```python
from build123d import *

# Parameters (mm, degrees)
SKETCH55_R               = 37
BOSS_EXTRUDE17_DEPTH     = 8
SKETCH56_R               = 37
SKETCH56_R_2             = 30
SKETCH56_R_3             = 28.8
CUT_EXTRUDE20_DEPTH      = 6
CUT_EXTRUDE21_DEPTH      = 5.5
FILLET1_R                = 0.5
FILLET2_R                = 2
BOSS_EXTRUDE18_START     = 6
BOSS_EXTRUDE18_DEPTH     = 6
CIRPATTERN1_COUNT        = 3
FILLET1_OF_CIRPATTERN1_R = 0.5
FILLET2_OF_CIRPATTERN1_R = 2


with BuildPart() as part:
    # Sketch55 → Boss-Extrude17 (new body)
    with BuildSketch(Plane.XY):
        Circle(SKETCH55_R)
        Polygon((-15.131119551888249, 22.33533974306702), (-25.90504070234881, -7.604599443277265), (-0.7697350404796751, -26.883764916532357), (25.354620105449243, -9.123888866834614), (16.52740298769779, 21.24243055544057), align=None, mode=Mode.SUBTRACT)
    extrude(amount=-BOSS_EXTRUDE17_DEPTH)

    # Sketch56 → Cut-Extrude20 (cut)
    # profile 1 of 2: a face of its own
    with BuildSketch(Plane.XY):
        Circle(SKETCH56_R)
        Circle(SKETCH56_R_2, mode=Mode.SUBTRACT)
    # profile 2 of 2: a face of its own
    with BuildSketch(Plane.XY):
        Circle(SKETCH56_R_3)
    extrude(amount=-CUT_EXTRUDE20_DEPTH, mode=Mode.SUBTRACT)

    # Sweep1: sweep along a path in Sketch58
    with BuildLine(Plane.XY.offset(-1)) as sweep1_path:
        ThreePointArc((32.05951496825865, -3.5), (32.25, 0), (32.05951496825865, 3.5))
    # Sketch59 → Sweep1 (sweep)
    with BuildSketch(Plane(origin=(0, 0, 0), x_dir=(1, 0, 0), z_dir=(0, 1, 0))):
        Polygon((32, 1.0000000000000009), (32, 4.6), (30, 5.25), (30, 1.0000000000000009), align=None)
    sweep1 = sweep(path=sweep1_path.line)

    # Sketch60 → Cut-Extrude21 (cut)
    with BuildSketch(Plane.XY):
        with BuildLine():
            Line((29.691011106511933, 4.294631471149185), (28.503370662251456, 4.122846212303217))
            ThreePointArc((28.503370662251456, 4.122846212303217), (28.570983048615947, 3.624765873225473), (28.629892436770504, 3.125581395348848))
            Line((28.629892436770504, 3.125581395348848), (29.822804621635946, 3.255813953488383))
            ThreePointArc((29.822804621635946, 3.255813953488383), (29.761440675641612, 3.7757977846098676), (29.691011106511933, 4.294631471149185))
        make_face()
        with BuildLine():
            Line((29.822804621635946, -3.255813953488384), (28.629892436770504, -3.1255813953488487))
            ThreePointArc((28.629892436770504, -3.1255813953488487), (28.57098304861595, -3.6247658732254733), (28.503370662251456, -4.122846212303217))
            Line((28.503370662251456, -4.122846212303217), (29.691011106511933, -4.294631471149185))
            ThreePointArc((29.691011106511933, -4.294631471149185), (29.761440675641612, -3.7757977846098676), (29.822804621635946, -3.255813953488384))
        make_face()
    cut_extrude21 = extrude(amount=-CUT_EXTRUDE21_DEPTH, mode=Mode.SUBTRACT)

    # Fillet1
    fillet1_edges = [part.edges().sort_by_distance(p)[0] for p in [
        (31.810991596411686, 3.472868217054266, -2.8000000000000003),
    ]]
    fillet(fillet1_edges, radius=FILLET1_R)

    # Fillet2
    fillet2_edges = [part.edges().sort_by_distance(p)[0] for p in [
        (31.810991596411686, -3.4728682170542657, -2.8000000000000003),
    ]]
    fillet(fillet2_edges, radius=FILLET2_R)

    # Sketch62 → Boss-Extrude18 (add)
    with BuildSketch(Plane.XY.offset(-6).offset(BOSS_EXTRUDE18_START)):
        with BuildLine():
            Line((35.035393105684086, 5.067665135956038), (28.225251300389694, 5.724961923877751))
            ThreePointArc((28.225251300389694, 5.724961923877751), (28.092883468127496, 6.342704348005581), (27.946997326196957, 6.957394659607891))
            Line((27.946997326196957, 6.957394659607891), (34.836258824834346, 6.29246144915893))
            ThreePointArc((34.836258824834346, 6.29246144915893), (34.94119298731927, 5.680935893223171), (35.035393105684086, 5.067665135956038))
        make_face()
    boss_extrude18 = extrude(amount=-BOSS_EXTRUDE18_DEPTH)

    # CirPattern1: Sweep1, Cut-Extrude21, Boss-Extrude18 ×3 about axis
    cirpattern1_axis = Axis((-3.9e-16, -9.2e-16, 0), (0, 0, 1))
    add([sweep1.rotate(cirpattern1_axis, i * 360 / CIRPATTERN1_COUNT) for i in range(1, CIRPATTERN1_COUNT)])
    add([cut_extrude21.rotate(cirpattern1_axis, i * 360 / CIRPATTERN1_COUNT) for i in range(1, CIRPATTERN1_COUNT)], mode=Mode.SUBTRACT)
    add([boss_extrude18.rotate(cirpattern1_axis, i * 360 / CIRPATTERN1_COUNT) for i in range(1, CIRPATTERN1_COUNT)])

    # Fillet1 of CirPattern1
    fillet1_of_cirpattern1_edges = [part.edges().sort_by_distance(p)[0] for p in [
        (-18.9130878981704, 25.812692733538686, -2.8000000000000003),
        (-12.897903698241294, -29.28556095059294, -2.8000000000000003),
    ]]
    fillet(fillet1_of_cirpattern1_edges, radius=FILLET1_OF_CIRPATTERN1_R)

    # Fillet2 of CirPattern1
    fillet2_of_cirpattern1_edges = [part.edges().sort_by_distance(p)[0] for p in [
        (-12.897903698241274, 29.28556095059295, -2.8000000000000003),
        (-18.91308789817042, -25.81269273353867, -2.8000000000000003),
    ]]
    fillet(fillet2_of_cirpattern1_edges, radius=FILLET2_OF_CIRPATTERN1_R)


solid = part.part
```
Build history of the part. All positions in model axes, mm. A direction names the side the tool comes from. Give positions to 0.01 mm unless a question says otherwise; leave off trailing zeros. Loops run counter-clockwise (first coordinate to the right, second up) from the corner with the lowest first, then second, coordinate; pieces in that order, holes last. Notation, with made-up numbers: (11, -33) -> (16, -33) arc R18 cw to (16, -14) -> close; hole circle Ø3 at (24, 13.25). An arc over 180 degrees is marked (long way). One line per question, with ' | ' between items.
Q1. Cut at B-B, the plane y = 14. Write the cut outline in (x, z), plus the area to 3 significant figures.
Filled sheet:
outline: (-34.25, -8) -> (-18.13, -8) -> (-18.13, -6) -> (-25.17, -6) -> (-25.17, 0) -> (-26.53, 0) -> (-26.53, -6) -> (-34.25, -6) -> close; (18.63, -8) -> (34.25, -8) -> (34.25, -6) -> (26.53, -6) -> (26.53, 0) -> (25.17, 0) -> (25.17, -6) -> (18.63, -6) -> close | area: 79.8 mm²
Q2. Cut at A-A, the plane x = 19. Write the cut outline in (y, z), plus the area to 3 significant figures.
Filled sheet:
outline: (-31.75, -8) -> (-13.44, -8) -> (-13.44, -6) -> (-21.64, -6) -> (-21.64, 0) -> (-23.22, 0) -> (-23.22, -6) -> (-31.75, -6) -> close; (12.74, -8) -> (31.75, -8) -> (31.75, -6) -> (23.22, -6) -> (23.22, 0) -> (21.64, 0) -> (21.64, -6) -> (12.74, -6) -> close | area: 93.5 mm²
Q3. Cut at C-C, the plane z = -3. Count the separate pieces of the cut face and the enclosed holes in it, plus the area to 3 significant figures.
Filled sheet:
separate pieces: 6 | enclosed holes: 0 | area: 272 mm²
Q4. Tool access for faces 1 (the flat face through (-10.3, -30.98, -2.96)), 2 (the flat face through (-21, 7, -6)), 3 (the flat face through (-21.68, 24.42, -2.96)): list every direction of +Z, -Z, +X, -X, +Y, -Y with a clear straight run to the whole face (end or side of a thin tool).
Filled sheet:
face 1: +Z, -Y | face 2: +Z | face 3: +Z, -X
Q5. Drill centre lines: line 1 along Y through (x, z) = (0, -3); line 2 along X through (y, z) = (0, -1.2); line 3 along X through (y, z) = (-7, -5.75). Where is each one in solid material? Low to high. Write a range as [from, to].
Filled sheet:
line 1: y = [-30, -28.8], [28.8, 30] | line 2: x = [-30, -28.8], [28.8, 32] | line 3: x = [-29.17, -27.94], [27.94, 29.17]
Q6. Drop flat-ended pins along their axis: pin 1 (1 mm diameter, centred on y = -17.5, z = -3, fed in from -X); pin 2 (2 mm diameter, centred on x = -16, y = 25.5, fed in from +Z); pin 3 (4 mm diameter, centred on x = 22, y = 26, fed in from +Z); pin 4 (3 mm diameter, centred on y = 17, z = -2.5, fed in from -X). Give the stop position or say it passes through.
Filled sheet:
pin 1: stops at x = -24.72 | pin 2: stops at z = 0 | pin 3: stops at z = -6 | pin 4: stops at x = -25.69
Q7. Cut at D-D, the plane y = 0. Write the cut outline in (x, z), plus the area to 3 significant figures.
Filled sheet:
outline: (-37, -8) -> (-23.17, -8) -> (-23.17, -6) -> (-28.8, -6) -> (-28.8, 0) -> (-30, 0) -> (-30, -6) -> (-37, -6) -> close; (22.7, -8) -> (37, -8) -> (37, -6) -> (30, -6) -> (30, -5.25) -> (32, -4.6) -> (32, -1) -> (30, -1) -> (30, 0) -> (28.8, 0) -> (28.8, -6) -> (22.7, -6) -> close | area: 78.5 mm²
